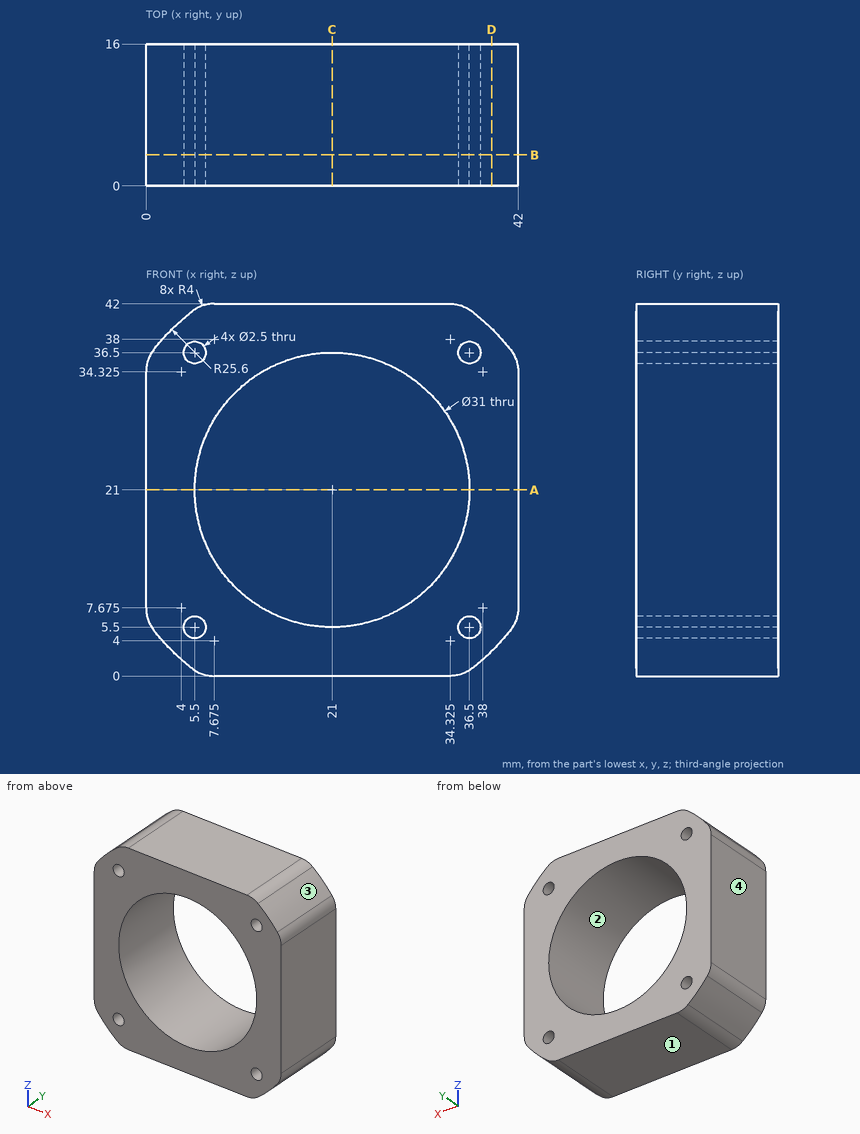
Check sheet for the drawn part. Datum: minimum x, y, z corner. Units: mm. Coordinates: 2 decimals unless noted, no trailing zeros. Order: outer loops, then holes, each group sorted by start corner. A loop starts at its lowest first (then second) coordinate and runs counter-clockwise, first axis right, second up. Notation, with made-up numbers: M 44.5,-22 L 78.5,-22 A31 cw 78.5,16 Z; hole C 61.25,1 d5. An arc over 180 degrees is marked long. One line per question, with ' | ' between items. Start each with the question number.
Item 1: Sectioned sample at D-D on x = 39. Record the cut outline in (y, z).
Item 2: Sectioned sample at A-A on z = 21. Record the cut outline in (x, y), and give its area (3 significant figures).
Item 3: Gauge pin test, flat end, axial feed: P1, Ø2, axis at x = 36.5, z = 5.5, coming from the -Y side. Record the tip position at first contact, or that the pin passes through.
Item 4: Mould release check, pull along X, two halves, no side actions. Record for the marked faces 1, 2, 3 and 4: pulls with the +X half, pulls with the -X half, needs draft (parallel to the pull), parting line crosses it, or undercut.
Item 5: Material ranges on line 1 (Z direction, x = 5, y = 13) (1 decimal); line 2 (X direction, y = 12.5, z = 20.5); line 3 (X direction, y = 14.75, z = 11), recorded low to high.
Item 6: Sectioned sample at C-C on x = 21. Record the cut outline in (y, z).
Item 7: Sectioned sample at B-B on y = 3.5. Count the separate pieces of the cut face and the enclosed holes in it, and give its area (3 significant figures).
Answer below:
1) outline: M 0,2.8 L 16,2.8 L 16,39.2 L 0,39.2 Z
2) outline: M 0,0 L 5.5,0 L 5.5,16 L 0,16 Z; M 36.5,0 L 42,0 L 42,16 L 36.5,16 Z | area: 176 mm^2
3) P1: passes through
4) face 1: needs draft | face 2: undercut | face 3: pulls with the +X half | face 4: pulls with the -X half
5) line 1: z = 1 to 4.4, 6.6 to 35.4, 37.6 to 41 | line 2: x = 0 to 5.51, 36.49 to 42 | line 3: x = 0 to 9.16, 32.84 to 42
6) outline: M 0,0 L 16,0 L 16,5.5 L 0,5.5 Z; M 0,36.5 L 16,36.5 L 16,42 L 0,42 Z
7) separate pieces: 1 | enclosed holes: 5 | area: 917 mm^2
